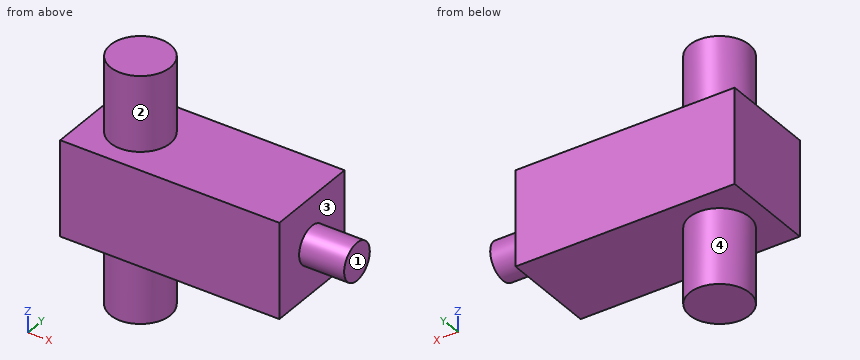
```python
from build123d import *

# Parameters (mm, degrees)
SKETCH1_W           = 29.2
SKETCH1_H           = 12.7
BOSS_EXTRUDE1_DEPTH = 12.7
SKETCH2_R           = 4
BOSS_EXTRUDE2_DEPTH = 10
SKETCH3_R           = 2.5
BOSS_EXTRUDE3_DEPTH = 6


with BuildPart() as part:
    # Sketch1 → Boss-Extrude1 (new body)
    with BuildSketch(Plane(origin=(0, 0, 0), x_dir=(1, 0, 0), z_dir=(0, 1, 0))):
        Rectangle(SKETCH1_W, SKETCH1_H)
    extrude(amount=BOSS_EXTRUDE1_DEPTH)

    # Sketch2 → Boss-Extrude2 (add)
    with BuildSketch(Plane.XY.offset(6.35)):
        with Locations(Location((-8.25, 6.35, 0), (0, 0, 180))):
            Circle(SKETCH2_R)
    boss_extrude2 = extrude(amount=BOSS_EXTRUDE2_DEPTH)

    # Mirror1: Boss-Extrude2 across plane
    add(boss_extrude2.mirror(Plane.XY))

    # Sketch3 → Boss-Extrude3 (add)
    with BuildSketch(Plane(origin=(14.6, 0, 0), x_dir=(0, 0, -1), z_dir=(1, 0, 0))):
        with Locations((0, 6.35)):
            Circle(SKETCH3_R)
    extrude(amount=BOSS_EXTRUDE3_DEPTH)


solid = part.part
```
Design review of the part built by this model. Coordinates are the model's own, in mm. Face numbers are marked on the shaded views. A direction names the side the tool comes from. Coordinates: 2 decimals unless noted, no trailing zeros. Loops run counter-clockwise (first coordinate to the right, second up) from the corner with the lowest first, then second, coordinate; pieces in that order, holes last. Notation, with made-up numbers: (48, 4) - (81, 4) arc R26 cw to (81, 26) - close; hole circle Ø8 at (-28, -25). An arc over 180 degrees is marked (long way). Use CSV: the item, a comma, the result in double quotes. Start each with the question number.
1) Consider section D-D on y = 12. Write out the cut boundary in (x, z), then the cut area to 3 significant figures.
2) Tool access review of the marked faces 1, 2, 3 and 4: name each direction out of +Z, -Z, +X, -X, +Y, -Y from which nothing blocks a thin tool from reaching the whole face with its end or side.
3) Consider section A-A on y = 6.35. Write out the cut boundary in (x, z).
4) For pin 1 Ø1.5 at (y, z) = (2, -10) entering from -X, flat-tipped, find the tip position at first contact; note if it passes through.
5) Consider section C-C on x = -8.25. Write out the cut boundary in (y, z), then the cut area to 3 significant figures.
6) Wall thickness on L1, parallel to Z at x = 13, y = 9.75; L2, parallel to X at y = 10.25, z = -1; L3, parallel to X at y = 4.5, z = -12: over which ranges is each line inside the solid? List them lowest first. Write a range as from..to.
7) Consider section B-B on z = 0. Write out the cut boundary in (x, y).
Geometry says:
1,outline,"(-14.6, -6.35) - (14.6, -6.35) - (14.6, 6.35) - (-14.6, 6.35) - close"
1,area,"371 mm^2"
2,face 1,"+Z, -Z, +X, +Y, -Y"
2,face 2,"+Z"
2,face 3,"+X"
2,face 4,"-Z"
3,outline,"(-14.6, -6.35) - (-12.25, -6.35) - (-12.25, -16.35) - (-4.25, -16.35) - (-4.25, -6.35) - (14.6, -6.35) - (14.6, -2.5) - (20.6, -2.5) - (20.6, 2.5) - (14.6, 2.5) - (14.6, 6.35) - (-4.25, 6.35) - (-4.25, 16.35) - (-12.25, 16.35) - (-12.25, 6.35) - (-14.6, 6.35) - close"
4,pin 1,"x = -9.99"
5,outline,"(0, -6.35) - (2.35, -6.35) - (2.35, -16.35) - (10.35, -16.35) - (10.35, -6.35) - (12.7, -6.35) - (12.7, 6.35) - (10.35, 6.35) - (10.35, 16.35) - (2.35, 16.35) - (2.35, 6.35) - (0, 6.35) - close"
5,area,"321 mm^2"
6,L1,"-6.35..6.35"
6,L2,"-14.6..14.6"
6,L3,"-11.8..-4.7"
7,outline,"(-14.6, 0) - (14.6, 0) - (14.6, 3.85) - (20.6, 3.85) - (20.6, 8.85) - (14.6, 8.85) - (14.6, 12.7) - (-14.6, 12.7) - close"
